from build123d import *

# Parameters (mm, degrees)
F1_DEPTH = 25
F3_D     = 6.5
F4_D     = 6.5
F5_R     = 8


with BuildPart() as f1:
    # F0 (on Top) → F1 (new body)
    with BuildSketch(Plane.XY):
        Polygon((31, 27.8544), (31, 32.8544), (12.5, 32.8544), (12.5, -3.2456), (0, -3.2456), (-12.5, -3.2456), (-12.5, 32.8544), (-31, 32.8544), (-31, 27.8544), (-17.5, 27.8544), (-17.5, -8.2456), (0, -8.2456), (17.5, -8.2456), (17.5, 27.8544), align=None)
    extrude(amount=F1_DEPTH)

    # F3 (through all)
    with Locations(Plane(origin=(0, 32.8544, 0), x_dir=(-1, 0, 0), z_dir=(0, 1, 0))):
        with Locations((25.023391, 12.5)):
            Hole(F3_D / 2)

    # F4 (through all)
    with Locations(Plane(origin=(0, 32.8544, 0), x_dir=(-1, 0, 0), z_dir=(0, 1, 0))):
        with Locations((-25.593, 12.5)):
            Hole(F4_D / 2)

    # F5
    f5_edges = [f1.edges().sort_by_distance(p)[0] for p in [
        (-31, 30.3544, 25),
        (-31, 30.3544, 0),
        (31, 30.3544, 25),
        (31, 30.3544, 0),
    ]]
    fillet(f5_edges, radius=F5_R)


solid = f1.part
Can you work these out from the model? Positions are in its coordinate system, mm. A direction names the side the tool comes from. Coordinates: 2 decimals unless noted, no trailing zeros. Loops run counter-clockwise (first coordinate to the right, second up) from the corner with the lowest first, then second, coordinate; pieces in that order, holes last. Notation, with made-up numbers: (-36.5, -32.5) - (-23.5, -32.5) arc R13 ccw to (-23.5, -24.5) - close; hole circle Ø9 at (-13.5, 65). An arc over 180 degrees is marked (long way). Answer as a JSON object with one key per item and string values. Group by question number.
Item 1: For pin 1 (15 mm diameter, centred on x = -21.5, z = 16, fed in from -Y); pin 2 (7.5 mm diameter, centred on y = 7.5, z = 16, fed in from +X); pin 3 (1 mm diameter, centred on y = 18.5, z = 15, fed in from -X); pin 4 (1 mm diameter, centred on x = -11, z = 19.5, fed in from +Y), each with a flat end and sliding along its axis, tell me the tip position at first contact or that it passes through.
Item 2: If we section it at D-D (x = 8.5): List the corners of the cut face in (y, z) for me.
Item 3: If we section it at C-C (z = 5.75): List the corners of the cut face in (x, y) for me.
Item 4: If I drill on L1, parallel to X at y = 14, z = 21.5; L2, parallel to Y at x = -28, z = 2.25; L3, parallel to Y at x = -8.5, z = 23.5, over which ranges is the centre line in solid material (lowest first)? Write a range as from..to.
Item 5: On a 3-axis mill with a long thin cutter (end or side, diameter ignored), from which of +Z, -Z, +X, -X, +Y, -Y can I reach the whole of each face in a straight line? I mean faces 1 (the face through (-17.5, 10, 12)), 2 (the face through (22, 32.854, 12)), 3 (the face through (-12.5, 15, 12)), 4 (the face through (17.5, 10, 12)), 5 (the face through (-28.594, 30.319, 22.719)). Say none if no direction works.
Item 6: If we section it at A-A (y = 13): List the corners of the cut face in (x, z) for me.
Item 7: If we mould it in two halves opening along X, with no side actions, what happens to faces 6 (the face through (-21.923, 30.319, 13.476)), 7 (the face through (31, 30, 12)), 8 (the face through (21, 27.854, 12))? For each: released by +X, released by -X, zero draft, split by the parting line, or undercut.
Item 8: If we section it at B-B (z = 12.5): List the corners of the cut face in (x, y) for me, plus the area to 3 significant figures.
Returned:
{
 "1": {"pin 1": "stops at y = -8.25", "pin 2": "stops at x = 17.5", "pin 3": "stops at x = -17.5", "pin 4": "stops at y = -3.25"},
 "2": {"outline": "(-8.25, 0) - (-3.25, 0) - (-3.25, 25) - (-8.25, 25) - close"},
 "3": {"outline": "(-30.68, 27.85) - (-17.5, 27.85) - (-17.5, -8.25) - (17.5, -8.25) - (17.5, 27.85) - (30.68, 27.85) - (30.68, 32.85) - (12.5, 32.85) - (12.5, -3.25) - (-12.5, -3.25) - (-12.5, 32.85) - (-30.68, 32.85) - close"},
 "4": {"L1": "x = -17.5..-12.5, 12.5..17.5", "L2": "y = 27.85..32.85", "L3": "y = -8.25..-3.25"},
 "5": {"face 1": "+Z, -Z, -X, -Y", "face 2": "+Z, -Z, +X, -X, +Y", "face 3": "+Z, -Z, +Y", "face 4": "+Z, -Z, +X, -Y", "face 5": "+Z, -X, +Y, -Y"},
 "6": {"outline": "(-17.5, 0) - (-12.5, 0) - (-12.5, 25) - (-17.5, 25) - close; (12.5, 0) - (17.5, 0) - (17.5, 25) - (12.5, 25) - close"},
 "7": {"face 6": "undercut", "face 7": "released by +X", "face 8": "zero draft"},
 "8": {"outline": "(-31, 27.85) - (-28.27, 27.85) - (-28.27, 32.85) - (-31, 32.85) - close; (-21.77, 27.85) - (-17.5, 27.85) - (-17.5, -8.25) - (17.5, -8.25) - (17.5, 27.85) - (22.34, 27.85) - (22.34, 32.85) - (12.5, 32.85) - (12.5, -3.25) - (-12.5, -3.25) - (-12.5, 32.85) - (-21.77, 32.85) - close; (28.84, 27.85) - (31, 27.85) - (31, 32.85) - (28.84, 32.85) - close", "area": "606 mm²"}
}
